For this review, take the finished solid that the model builds, in its own axes (mm). A direction names the side the tool comes from. Give positions to 0.01 mm unless a question says otherwise; leave off trailing zeros. Loops run counter-clockwise (first coordinate to the right, second up) from the corner with the lowest first, then second, coordinate; pieces in that order, holes last.
```python
from build123d import *

# Parameters (mm, degrees)
CUT_EXTRUDE_1_DEPTH = 7.44


with BuildPart() as part:
    # Sketch 1 → Revolve 1 (revolve)
    with BuildSketch(Plane.XY):
        with BuildLine():
            Line((0, 6), (-32.30531511, 6))
            ThreePointArc((-32.30531511, 6), (-32.539753787, 6.047697088), (-32.73691899, 6.183204978))
            Line((-32.73691899, 6.183204978), (-39.744724485, 13.44))
            Line((-39.744724485, 13.44), (-40, 13.44))
            Line((-40, 13.44), (-40, 0))
            Line((-40, 0), (0, 0))
            Line((0, 0), (0, 6))
        make_face()
    revolve(axis=Axis((0, 0, 0), (-1, 0, 0)))

    # Sketch 2 → Cut-Extrude 1 (cut)
    with BuildSketch(Plane.ZY.offset(40)):
        Polygon((0, 4.618802154), (-4, 2.309401077), (-4, -2.309401077), (0, -4.618802154), (4, -2.309401077), (4, 2.309401077), align=None)
    extrude(amount=-CUT_EXTRUDE_1_DEPTH, mode=Mode.SUBTRACT)

    # Sketch 6 → Revolve 2 (revolve)
    with BuildSketch(Plane.XY, mode=Mode.PRIVATE) as revolve_2_sk:
        Polygon((-35.7, 4.618802154), (-33.033333333, 0), (-31.41, 0), (-31.41, 4.618802154), align=None)
    revolve(revolve_2_sk.sketch.rotate(Axis((-40, 0, 0), (1, 0, 0)), 90), axis=Axis((-40, 0, 0), (1, 0, 0)))

    # Sketch 7 → Cut-Revolve 2 (revolve, cut)
    with BuildSketch(Plane.XY, mode=Mode.PRIVATE) as cut_revolve_2_sk:
        Polygon((-40, 4.618802154), (-40, 0), (-38.85, 0), align=None)
    revolve(cut_revolve_2_sk.sketch.rotate(Axis((-40, 0, 0), (1, 0, 0)), 90), axis=Axis((-40, 0, 0), (1, 0, 0)), mode=Mode.SUBTRACT)

    # Sketch 4 → Cut-Revolve 1 (revolve, cut)
    with BuildSketch(Plane.XY, mode=Mode.PRIVATE) as cut_revolve_1_sk:
        Polygon((-0.875, 6), (0, 4.484455543), (0.875, 6), align=None)
    revolve(cut_revolve_1_sk.sketch.rotate(Axis((-0.875, 0, 0), (1, 0, 0)), 90), axis=Axis((-0.875, 0, 0), (1, 0, 0)), mode=Mode.SUBTRACT)


solid = part.part
```
Item 1: Tool access review of faces 1 (the conical face through (-39.907, -3.692, -2.095)), 2 (the flat face through (0, 0, 0)): name each direction out of +Z, -Z, +X, -X, +Y, -Y from which nothing blocks a thin tool from reaching the whole face with its end or side.
Answer:
face 1: -X
face 2: +Z, -Z, +X, +Y, -Y
Item 2: Clearance check with flat-ended pins moving along their axes: pin 1 Ø5 at (x, y) = (-38.5, 0.5) entering from +Z; pin 2 Ø4 at (x, y) = (-11.5, 3.5) entering from -Z; pin 3 Ø8 at (x, z) = (-35, -2) entering from +Y; pin 4 Ø12 at (x, z) = (-33, -9.5) entering from +Y. State where each tip first meets the part, or that it passes through.
Answer:
pin 1: stops at z = 13.44
pin 2: stops at z = -5.81
pin 3: stops at y = 12.55
pin 4: stops at y = 9.9
Item 3: The part is to be moulded in two halves that separate along Y. For faces 3 (the flat face through (-40, 0, 6)), 4 (the conical face through (-33.46, 0.45, -0.59)), 5 (the flat face through (-37.704, -3.448, -2.028)), 6 (the cylindrical face through (-16.81, 5.723, -1.802)), say which applies: released by +Y, released by -Y, zero draft, split by the parting line, or undercut.
Answer:
face 3: zero draft
face 4: undercut
face 5: undercut
face 6: split by the parting line
Item 4: For L1, parallel to Y at x = -36, z = -3; L2, parallel to Z at x = -36, y = 1; L3, parallel to Y at x = -4.5, z = 0, list the stretches that pass through material, from the lowest coordinate up.
Answer:
L1: y = -9.08 to -2.89, 2.89 to 9.08
L2: z = -9.51 to -4, 4 to 9.51
L3: y = -6 to 6
Item 5: Take a section at A-A on x = -19. Give the boundary of the cut face in (y, z), and give its area (3 significant figures).
Answer:
outline: circle Ø12 at (0, 0)
area: 113 mm2
